Read the model definition and answer for the solid it produces. Units are mm, in the model's axes. A direction names the side the tool comes from. Coordinates: 2 decimals unless noted, no trailing zeros. Loops run counter-clockwise (first coordinate to the right, second up) from the corner with the lowest first, then second, coordinate; pieces in that order, holes last. Notation, with made-up numbers: (62.25, 60) -> (79.25, 60) arc R36 ccw to (79.25, 99) -> close; hole circle Ø10 at (53.5, 24). An arc over 180 degrees is marked (long way). Answer as a JSON object with one key per item and string values. Group by question number.
1) Which of the six approach directions +Z, -Z, +X, -X, +Y, -Y give full straight-line access (tool end or side, diameter ignored) to faces 1 (the face through (0, -11.112, 21)), 2 (the face through (11.6, -0.3, 4.4))?
2) Section D-D, the plane z = 5.5 is taken. Give the vertices of the cut face in (x, y) (3 decimals).
3) Section A-A, the plane z = 20.75 is taken. Give the vertices of the cut face in (x, y), plus the area to 3 significant figures.
4) Section C-C, the plane y = -6 is taken. Give the vertices of the cut face in (x, z).
5) Determine the mould class of faces 3 (the face through (0.178, 0.267, 0.743)), 4 (the face through (0, 15, 25.4)), 5 (the face through (0, -19.05, 10)) for opening direction Y: released by +Y, released by -Y, zero draft, split by the parting line, or undercut.
6) Consider probe 1 along Y at (x, z) = (-7, 22.25); probe 2 along Y at (x, z) = (7.25, 7.5); probe 3 along Z at (x, y) = (-5.25, -17). Determine where each line is inside the solid, lowest interval first. Write a range as [from, to].
7) Flat-ended cylindrical pins translate along their axes: P1, Ø2, axis at y = -14, z = 8, coming from the -X side; P2, Ø1, axis at x = -7.5, y = 1, coming from the -Z side; P3, Ø6, axis at y = -13.5, z = 18.5, coming from the -X side (3 decimals). Find the tip coordinate at first contact, or state that the pin passes through.
from build123d import *

# Parameters (mm, degrees)
F1_DEPTH  = 19.05
F1_FACE_W = 25.4
F1_FACE_H = 25.4
F2_DEPTH  = 19.05
F4_DEPTH  = 25.4
F6_DEPTH  = 25.4
F8_DEPTH  = 38.1


with BuildPart() as f1:
    # F0 (on Front) → F1 (new body)
    with BuildSketch(Plane.XZ):
        Polygon((-12.7, 0), (0, 0), (12.7, 0), (12.7, 25.4), (-12.7, 25.4), align=None)
    extrude(amount=F1_DEPTH)

    # F1_face (on face) → F2 (join)
    with BuildSketch(Plane(origin=(0, 0, 12.7), x_dir=(1, 0, 0), z_dir=(0, 1, 0))):
        Rectangle(F1_FACE_W, F1_FACE_H)
    extrude(amount=F2_DEPTH)

    # F3 (on face) → F4 (cut)
    with BuildSketch(Plane.YZ.offset(12.7)):
        with BuildLine():
            Line((-19.05, 0), (19.05, 0))
            ThreePointArc((19.05, 0), (0, 0.743338), (-19.05, 0))
        make_face()
    extrude(amount=-F4_DEPTH, mode=Mode.SUBTRACT)

    # F5 (on face) → F6 (cut)
    with BuildSketch(Plane.YZ.offset(12.7)):
        with BuildLine():
            Line((-11.1125, 25.4), (-11.1125, 15.875))
            ThreePointArc((-11.1125, 15.875), (0, 4.7625), (11.1125, 15.875))
            Line((11.1125, 15.875), (11.1125, 25.4))
            Line((11.1125, 25.4), (-11.1125, 25.4))
        make_face()
    extrude(amount=-F6_DEPTH, mode=Mode.SUBTRACT)

    # F7 (on face) → F8 (cut)
    with BuildSketch(Plane.XZ.offset(19.05)):
        Polygon((-12.7, 25.4), (-12.7, 0), (-6.35, 25.4), align=None)
        Polygon((6.35, 25.4), (12.7, 0), (12.7, 25.4), align=None)
    extrude(amount=-F8_DEPTH, mode=Mode.SUBTRACT)


solid = f1.part
Determined:
{
 "1": {"face 1": "+Z, +X, -X", "face 2": "+Z, +X, +Y, -Y"},
 "2": {"outline": "(-11.325, -19.05) -> (11.325, -19.05) -> (11.325, -3.981) -> (-11.325, -3.981) -> close; (-11.325, 3.981) -> (11.325, 3.981) -> (11.325, 19.05) -> (-11.325, 19.05) -> close"},
 "3": {"outline": "(-7.51, -19.05) -> (7.51, -19.05) -> (7.51, -11.11) -> (-7.51, -11.11) -> close; (-7.51, 11.11) -> (7.51, 11.11) -> (7.51, 19.05) -> (-7.51, 19.05) -> close", "area": "239 mm²"},
 "4": {"outline": "(-12.53, 0.67) -> (12.53, 0.67) -> (11.07, 6.52) -> (-11.07, 6.52) -> close"},
 "5": {"face 3": "undercut", "face 4": "zero draft", "face 5": "released by -Y"},
 "6": {"probe 1": "[-19.05, -11.11], [11.11, 19.05]", "probe 2": "[-19.05, -7.3], [7.3, 19.05]", "probe 3": "[0.15, 25.4]"},
 "7": {"P1": "x = -10.95", "P2": "z = 0.74", "P3": "x = -8.825"}
}
